Verification items for the finished model (mm, model axes). A direction names the side the tool comes from. Coordinates: 2 decimals unless noted, no trailing zeros. Order: outer loops, then holes, each group sorted by start corner. A loop starts at its lowest first (then second) coordinate and runs counter-clockwise, first axis right, second up. Notation, with made-up numbers: M -39,-18.75 L -8,-18.75 A21 ccw -8,5.25 Z; hole C 50,-21 d4. An arc over 180 degrees is marked long. Answer as a JSON object with one key per item and string values. Group by question number.
(1) Mould release check, pull along X, two halves, no side actions. Record for faces 1 (the face through (-21.79, 4, 2.05)), 2 (the face through (38.1, 0, 0)), 3 (the face through (0.53, -1.36, -8.2)): released by +X, released by -X, zero draft, split by the parting line, or undercut.
(2) Access from +Z, -Z, +X, -X, +Y, -Y to the whole of each face (thin tool, end or side, straight path). Record for faces 4 (the face through (0.53, 1.32, -8.16)), 5 (the face through (-25, 4, -4.15)), 6 (the face through (11.05, -0.09, 0.04)).
(3) Cross-section at D-D (x = 11.5). Enter the section's corners in (y, z) (3 decimals).
(4) Material ranges on line 1 (Z direction, x = 24.5, y = 2.75) (3 decimals); line 2 (X direction, y = -2, z = 0); line 3 (Y direction, x = -27.5, z = 2), recorded low to high.
(5) Cross-section at B-B (y = 3.75). Enter the section's corners in (x, z) (3 decimals).
(6) Cross-section at C-C (x = -10). Enter the section's corners in (y, z) (3 decimals), plus the area to 3 significant figures.
(7) Gauge pin test, flat ends, axial feed: pin 1 Ø4 at (x, z) = (25.4, 0) entering from +Y; pin 2 Ø6 at (x, z) = (-25.4, 0) entering from +Y. Record the tip position at first contact, or that the pin passes through.
Autodesk Inventor part; units mm, degrees
ref_plane "YZ Plane" through (0, 0, 0) normal (1, 0, 0) x (0, 1, 0)
ref_plane "XZ Plane" through (0, 0, 0) normal (0, 1, 0) x (-1, 0, 0)
ref_plane "XY Plane" through (0, 0, 0) normal (0, 0, 1) x (1, 0, 0)
sketch "Sketch1" plane through (0, 0, 0) normal (0, 1, 0) x (-1, 0, 0)
  line L0 (-38.1, 9.525) -> (38.1, 9.525)
  line L1 (38.1, 9.525) -> (38.1, -9.525)
  line L2 (38.1, -9.525) -> (-38.1, -9.525)
  line L3 (-38.1, -9.525) -> (-38.1, 9.525)
  line L4 (-38.1, 9.525) -> (38.1, -9.525) construction
  line L5 (38.1, 9.525) -> (-38.1, -9.525) construction
  point P0 (0, 0)
  dimension "d0" = 76.2
  dimension "d1" = 19.05
extrude "Extrusion1" add sketch "Sketch1" along normal mid plane 12.7
sketch "Sketch2" plane through (38.1, -6.35, -9.525) normal (1, 0, 0) x (0, 0, -1)
  line L0 (0, 3.663) -> (-2.687, 6.35)
  line L1 (-2.687, 6.35) -> (0, 9.037)
  line L2 (0, 9.037) -> (2.687, 6.35)
  line L3 (2.687, 6.35) -> (0, 3.663)
  line L4 (-19.05, 12.7) -> (0, 12.7)
  line L5 (0, 12.7) -> (0, 0)
  point P0 (-9.525, 6.35)
  point P1 (0, 6.35)
  dimension "d4" = 45
  dimension "d5" = 3.8
extrude "Extrusion2" cut sketch "Sketch2" against normal through all
sketch "Sketch5" plane through (0, 6.35, 0) normal (0, 1, 0) x (1, 0, 0)
  line L0 (-38.1, 9.525) -> (-38.1, -9.525)
  line L1 (38.1, -9.525) -> (38.1, 9.525)
  point P0 (0, 0)
  point P1 (-25.4, 0)
  point P2 (25.4, 0)
  dimension "d18" = 12.7
  dimension "d19" = 12.7
hole "Hole1" at (-25.4, 6.35, 0) at (25.4, 6.35, 0) direction (0, -1, 0) diameter 5.3086 end through all
sketch "Sketch6" plane through (0, 6.35, 0) normal (0, 1, 0) x (1, 0, 0)
  line L0 (-38.1, 9.525) -> (-38.1, -9.525)
  line L1 (38.1, -9.525) -> (38.1, 9.525)
  line L2 (-38.1, -9.525) -> (38.1, -9.525)
  line L3 (38.1, 6.838) -> (-38.1, 6.838)
  circle A0 centre (-25.4, 0) radius 2.6543
  point P0 (0, 0)
  point P1 (-10, 2.5)
  point P2 (10, 2.5)
  dimension "d27" = 28.1
  dimension "d28" = 28.1
  dimension "d38" = 2.5
hole "Hole2" at (-10, 6.35, -2.5) at (10, 6.35, -2.5) direction (0, -1, 0) diameter 5.5 end through all
sketch "Sketch7" plane through (0, 6.35, 0) normal (0, 1, 0) x (1, 0, 0)
  circle A0 centre (-25.4, 0) radius 2.6543
  circle A1 centre (25.4, 0) radius 2.6543
  line L0 (-23.004, 4.15) -> (-20.608, 0)
  line L1 (-20.608, 0) -> (-23.004, -4.15)
  line L2 (-23.004, -4.15) -> (-27.796, -4.15)
  line L3 (-27.796, -4.15) -> (-30.192, 0)
  line L4 (-30.192, 0) -> (-27.796, 4.15)
  line L5 (-27.796, 4.15) -> (-23.004, 4.15)
  line L6 (23.004, -4.15) -> (20.608, 0)
  line L7 (20.608, 0) -> (23.004, 4.15)
  line L8 (23.004, 4.15) -> (27.796, 4.15)
  line L9 (27.796, 4.15) -> (30.192, 0)
  line L10 (30.192, 0) -> (27.796, -4.15)
  line L11 (27.796, -4.15) -> (23.004, -4.15)
  point P0 (0, 0)
  dimension "d39" = 8.3
  dimension "d40" = 8.3
extrude "Extrusion5" cut sketch "Sketch7" against normal blind 4.7625 contours A1 | L0 L1 L2 L3 L4 L5 | L6 L7 L8 L9 L10 L11
equation "\"d40\" = d39"
properties part number "X-Axis_Mount_Slide_LM3005" material "Acetal Resin, White"
Taken from the geometry:
{
 "1": {"face 1": "undercut", "face 2": "released by +X", "face 3": "zero draft"},
 "2": {"face 4": "-Z, +X, -X", "face 5": "+Y", "face 6": "+Y, -Y"},
 "3": {"outline": "M -6.35,-9.525 L -2.687,-9.525 L 0,-6.838 L 2.687,-9.525 L 6.35,-9.525 L 6.35,-4.805 L -6.35,-4.805 Z; M -6.35,-0.195 L 6.35,-0.195 L 6.35,9.525 L -6.35,9.525 Z"},
 "4": {"line 1": "z = -9.525 to -4.15, 4.15 to 9.525", "line 2": "x = -38.1 to -28.05, -22.75 to -11.15, -8.85 to 8.85, 11.15 to 22.75, 28.05 to 38.1", "line 3": "y = -6.35 to 1.59"},
 "5": {"outline": "M -38.1,-9.525 L 38.1,-9.525 L 38.1,9.525 L -38.1,9.525 Z; hole M -30.192,0 L -27.796,-4.15 L -23.004,-4.15 L -20.608,0 L -23.004,4.15 L -27.796,4.15 Z; hole C -10,-2.5 d5.5; hole C 10,-2.5 d5.5; hole M 20.608,0 L 23.004,-4.15 L 27.796,-4.15 L 30.192,0 L 27.796,4.15 L 23.004,4.15 Z"},
 "6": {"outline": "M -6.35,-9.525 L -2.687,-9.525 L 0,-6.838 L 2.687,-9.525 L 6.35,-9.525 L 6.35,-5.25 L -6.35,-5.25 Z; M -6.35,0.25 L 6.35,0.25 L 6.35,9.525 L -6.35,9.525 Z", "area": "165 mm²"},
 "7": {"pin 1": "passes through", "pin 2": "stops at y = 1.59"}
}
